Drawing for the job (mm, zero at the part's lowest x, y, z). A direction names the side the tool comes from. Give positions to 0.01 mm unless a question says otherwise; leave off trailing zeros. Order: outer loops, then holes, each group sorted by start corner. A loop starts at its lowest first (then second) coordinate and runs counter-clockwise, first axis right, second up. Notation, with made-up numbers: M -26,49.25 L 24,49.25 A19 cw 24,54.25 Z; hole C 88.5,-29.5 d10. An arc over 180 degrees is marked long. Answer as a JSON object with one key per item and string values.
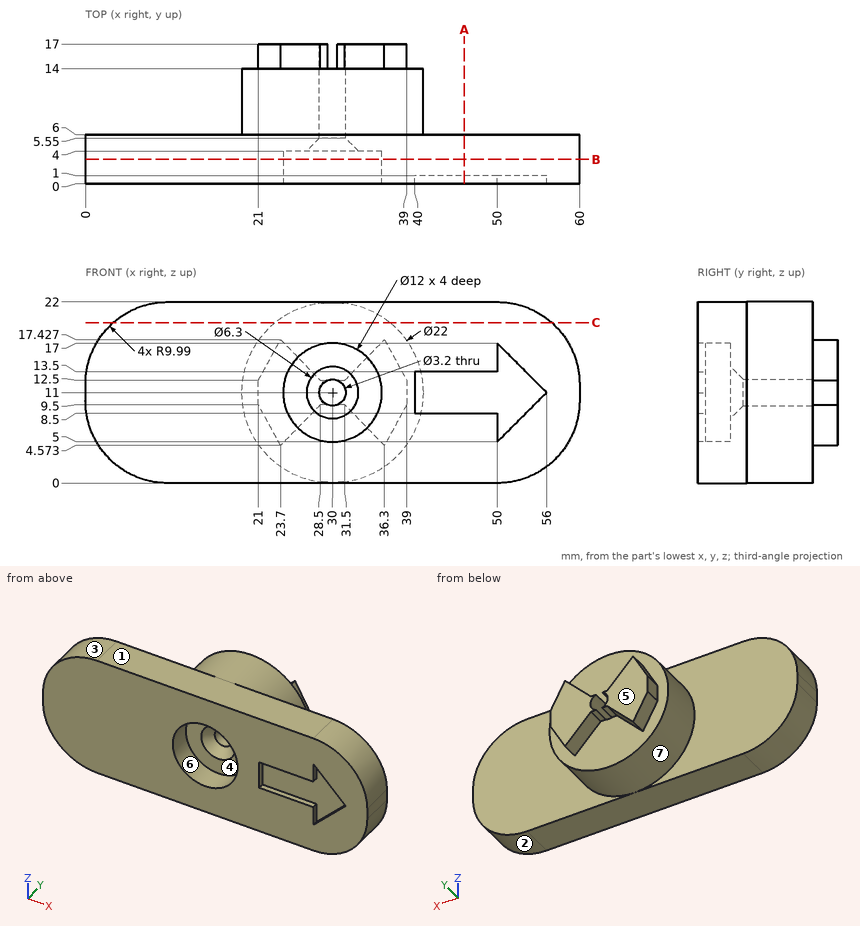
1. Which spindle directions (+Z, -Z, +X, -X, +Y, -Y) get a long thin tool onto all of the face, cutting with end or side? Do the marked faces 5, 6 and 7. Say none if no direction does.
Worked answers:
{"face 5": "+Z, -Z, +X, -X, +Y", "face 6": "-Y", "face 7": "+Y"}
2. Cut at C-C on z = 19.5. Give the cut face in (x, y).
Worked answers:
{"outline": "M 3.38,0 L 56.62,0 L 56.62,6 L 36.98,6 L 36.98,14 L 23.02,14 L 23.02,6 L 3.38,6 Z"}
3. Cut at A-A on x = 46. Give the cut face in (y, z), plus the area to 3 significant figures.
Worked answers:
{"outline": "M 0,0 L 6,0 L 6,22 L 0,22 L 0,13.5 L 1,13.5 L 1,8.5 L 0,8.5 Z", "area": "127 mm^2"}
4. Probe line 1 along Z through (x, y) = (30, 2.8); line 2 along X through (y, z) = (13.5, 11); line 3 along Y through (x, z) = (28.5, 17). List the from-to ranges inside material, lowest first.
Worked answers:
{"line 1": "z = 0 to 5, 17 to 22", "line 2": "x = 19 to 28.4, 31.6 to 41", "line 3": "y = 0 to 14"}
5. Cut at B-B on y = 3. Give the cut face in (x, z).
Worked answers:
{"outline": "M 0,9.99 A9.99 ccw 9.99,0 L 50.01,0 A9.99 ccw 60,9.99 L 60,12.01 A9.99 ccw 50.01,22 L 9.99,22 A9.99 ccw 0,12.01 Z; hole C 30,11 d12"}
6. Two-plate mould, pull along X, no slides. Class the marked faces 1, 2, 3 and 4: +X half, -X half, draft (parallel to the pull), parting line (faces both ways), or undercut.
Worked answers:
{"face 1": "draft", "face 2": "+X half", "face 3": "-X half", "face 4": "undercut"}
7. Pin check, flat tips, straight feed: P1, Ø4, axis at x = 36, y = 9.5, coming from the -Z side; P2, Ø5, axis at y = 5, z = 19, coming from the +X side (1 decimal); P3, Ø0.8, axis at y = 0.5, z = 14.5, coming from the +X side; P4, Ø1.9, axis at x = 30, z = 11, coming from the +Y side. Stop position of each tip, or through.
Worked answers:
{"P1": "stops at z = 0.75", "P2": "stops at x = 58.9", "P3": "stops at x = 59.78", "P4": "passes through"}
